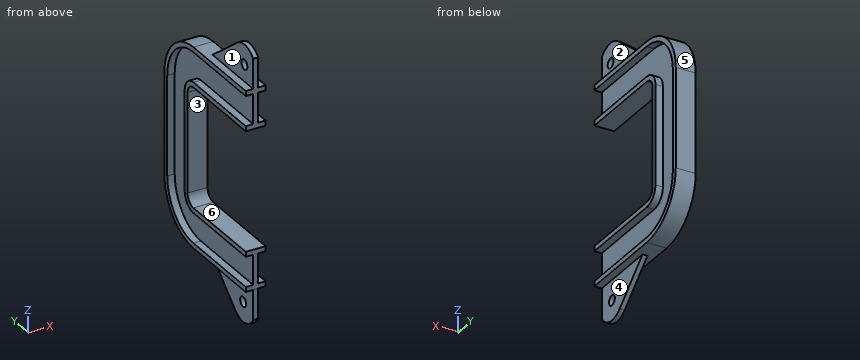
from build123d import *

# Parameters (mm, degrees)
F4_DEPTH  = 2.5
F5_R      = 5
F6_DEPTH  = 25.4
F8_DEPTH  = 2.5
F9_R      = 5
F10_DEPTH = 25.4


with BuildPart() as f2:
    # F2: sweep along a path in F1
    with BuildLine(Plane.YZ) as f2_path:
        Line((0, 60), (90, 60))
        ThreePointArc((90, 60), (97.071068, 57.071068), (100, 50))
        Line((100, 50), (100, -50))
        ThreePointArc((100, -50), (97.071068, -57.071068), (90, -60))
        Line((90, -60), (0, -60))
    # F0 (on Front) → F2 (sweep)
    with BuildSketch(Plane.XZ):
        Polygon((-10, 60), (0, 60), (10, 60), (10, 65), (2.5, 65), (2.5, 95), (10, 95), (10, 100), (0, 100), (-10, 100), (-10, 95), (-2.5, 95), (-2.5, 65), (-10, 65), align=None)
    sweep(path=f2_path.line)

    # F3 (on Right) → F4 (join, symmetric)
    with BuildSketch(Plane.YZ):
        with BuildLine():
            Line((0, 130), (0, 100))
            Line((0, 100), (70, 100))
            Line((70, 100), (27.347526, 132.802719))
            ThreePointArc((27.347526, 132.802719), (13.115891, 136.844791), (0, 130))
        make_face()
    extrude(amount=F4_DEPTH, both=True)

    # F5 (on face) → F6 (cut)
    with BuildSketch(Plane(origin=(-2.5, 0, 0), x_dir=(0, -1, 0), z_dir=(-1, 0, 0))):
        with Locations((-15.154916, 116.949004)):
            Circle(F5_R)
    extrude(amount=-F6_DEPTH, mode=Mode.SUBTRACT)

    # F7 (on Right) → F8 (join, symmetric)
    with BuildSketch(Plane.YZ):
        with BuildLine():
            Line((70, -100), (0, -100))
            Line((0, -100), (0, -130))
            ThreePointArc((0, -130), (14.162499, -139.933551), (30.774234, -135.106332))
            Line((30.774234, -135.106332), (70, -100))
        make_face()
    extrude(amount=F8_DEPTH, both=True)

    # F9 (on face) → F10 (cut)
    with BuildSketch(Plane.YZ.offset(2.5)):
        with Locations((17.436313, -120.203317)):
            Circle(F9_R)
    extrude(amount=-F10_DEPTH, mode=Mode.SUBTRACT)


solid = f2.part
Source: CAD feature listing. Evaluate the final solid. Frame: model axes, mm. Face numbers are marked on the shaded views. A direction names the side the tool comes from. Round coordinates to 2 decimals unless told otherwise and drop trailing zeros. Order: outer loops, then holes, each group sorted by start corner. A loop starts at its lowest first (then second) coordinate and runs counter-clockwise, first axis right, second up. Notation, with made-up numbers: (21, -11) - (59, -11) arc R20 cw to (59, 24) - close; hole circle Ø5 at (-30.5, -10.5). An arc over 180 degrees is marked (long way). Use a Markdown table: item, result. Add a question column.
1. Section query A-A (y = 83.5). Return the cut outline in (x, z).
2. Section query C-C (z = 23). Return the cut outline in (x, y).
3. Section query B-B (x = 5.5). Return the cut outline in (y, z), then the cut area to 3 significant figures.
4. Line query: probe 1 along Z at (x, y) = (2.75, 12); probe 2 along Y at (x, z) = (7.75, 22.5); probe 3 along Z at (x, y) = (3.75, 100.5). Output: solid intervals per line, ascending.
5. Mould query, pull axis Z, two halves, no side actions, for the marked faces 4, 5 and 6. Classes: +Z half, -Z half, draft (parallel to the pull), parting line (faces both ways), or undercut.
6. Set-up query: the marked faces 1, 2 and 3. Return all of +Z, -Z, +X, -X, +Y, -Y with unobstructed straight access to the full face (end or side cutting, diameter ignored); none if empty.
7. Section query D-D (y = 118). Return the cut outline in (x, z).
8. First-contact query: pin 1 (12 mm diameter, centred on x = -2, y = 111, fed in from -Z); pin 2 (5 mm diameter, centred on y = 56.5, z = -82.5, fed in from +X); pin 3 (4 mm diameter, centred on x = 7, z = -3.5, fed in from -Y); pin 4 (9 mm diameter, centred on y = 17.44, z = -120.2, fed in from +X). Flat tips, straight axial feed; report the tip coordinate or a pass-through.
Derived:
| question | item | result |
|---|---|---|
| 1 | outline | (-10, -100) - (10, -100) - (10, -95) - (2.5, -95) - (2.5, -65) - (10, -65) - (10, -60) - (-10, -60) - (-10, -65) - (-2.5, -65) - (-2.5, -95) - (-10, -95) - close; (-10, 60) - (10, 60) - (10, 65) - (2.5, 65) - (2.5, 95) - (10, 95) - (10, 100) - (-10, 100) - (-10, 95) - (-2.5, 95) - (-2.5, 65) - (-10, 65) - close |
| 2 | outline | (-10, 100) - (10, 100) - (10, 105) - (2.5, 105) - (2.5, 135) - (10, 135) - (10, 140) - (-10, 140) - (-10, 135) - (-2.5, 135) - (-2.5, 105) - (-10, 105) - close |
| 3 | outline | (0, -100) - (90, -100) arc R50 ccw to (140, -50) - (140, 50) arc R50 ccw to (90, 100) - (0, 100) - (0, 95) - (90, 95) arc R45 cw to (135, 50) - (135, -50) arc R45 cw to (90, -95) - (0, -95) - close; (0, -65) - (90, -65) arc R15 ccw to (105, -50) - (105, 50) arc R15 ccw to (90, 65) - (0, 65) - (0, 60) - (90, 60) arc R10 cw to (100, 50) - (100, -50) arc R10 cw to (90, -60) - (0, -60) - close |
| 3 | area | 3,740 mm2 |
| 4 | probe 1 | -100 to -95, -65 to -60, 60 to 65, 95 to 100 |
| 4 | probe 2 | 100 to 105, 135 to 140 |
| 4 | probe 3 | -98.89 to -93.76, -60.71 to 60.71, 93.76 to 98.89 |
| 5 | face 4 | draft |
| 5 | face 5 | +Z half |
| 5 | face 6 | undercut |
| 6 | face 1 | +Z, -X, +Y, -Y |
| 6 | face 2 | +Z, +X, +Y, -Y |
| 6 | face 3 | +X, -X, -Y |
| 7 | outline | (-10, -91.42) - (10, -91.42) - (10, -85.23) - (2.5, -85.23) - (2.5, 85.23) - (10, 85.23) - (10, 91.42) - (-10, 91.42) - (-10, 85.23) - (-2.5, 85.23) - (-2.5, -85.23) - (-10, -85.23) - close |
| 8 | pin 1 | z = -97.7 |
| 8 | pin 2 | x = 2.5 |
| 8 | pin 3 | y = 100 |
| 8 | pin 4 | through |
